```python
from build123d import *

# Parameters (mm, degrees)
SKETCH1_R              = 39
BOSS_EXTRUDE1_DEPTH    = 8
SKETCH2_R              = 8
BOSS_EXTRUDE2_DEPTH    = 10
SKETCH3_R              = 3
CUT_EXTRUDE1_DEPTH     = 59.017238817
M5_TAPPED_HOLE1_REACH  = 64.446
M5_TAPPED_HOLE1_BORE_R = 2.1
SKETCH5_W              = 8
SKETCH5_H              = 5


with BuildPart() as part:
    # Sketch1 → Boss-Extrude1 (new body)
    with BuildSketch(Plane.XY):
        Circle(SKETCH1_R)
    extrude(amount=BOSS_EXTRUDE1_DEPTH)

    # Sketch2 → Boss-Extrude2 (add)
    with BuildSketch(Plane.XY.offset(8)):
        Circle(SKETCH2_R)
    extrude(amount=BOSS_EXTRUDE2_DEPTH)

    # Sketch3 → Cut-Extrude1 (cut, through all)
    with BuildSketch(Plane.XY.offset(18)):
        Circle(SKETCH3_R)
    extrude(amount=-CUT_EXTRUDE1_DEPTH, mode=Mode.SUBTRACT)

    # M5 Tapped Hole1 bore (on position points) → M5 Tapped Hole1 (cut, up to next)
    with BuildSketch(Plane(origin=(-0.006341918, 7.999997486, 13), x_dir=(0.999999685782, 0.000792739743, 0), z_dir=(-0.000792739743, 0.999999685782, 0)), mode=Mode.PRIVATE) as m5_tapped_hole1_sk1:
        Circle(M5_TAPPED_HOLE1_BORE_R)
    m5_tapped_hole1_tool1 = extrude(m5_tapped_hole1_sk1.sketch, amount=-M5_TAPPED_HOLE1_REACH, mode=Mode.PRIVATE) & part.part
    add(m5_tapped_hole1_tool1.solids().sort_by_distance((-0.006342, 7.999997, 13))[0], mode=Mode.SUBTRACT)

    # Sketch5 → Cut-Revolve1 (revolve, cut)
    with BuildSketch(Plane(origin=(0, 0, 0), x_dir=(1, 0, 0), z_dir=(0, 1, 0))):
        with Locations((-39, -4)):
            Rectangle(SKETCH5_W, SKETCH5_H)
    revolve(axis=Axis((0, 0, 0), (0, 0, 1)), mode=Mode.SUBTRACT)


solid = part.part
```
Check sheet for the modelled part. Datum: model origin and axes. Units: mm. A direction names the side the tool comes from. Coordinates: 2 decimals unless noted, no trailing zeros. Loops run counter-clockwise (first coordinate to the right, second up) from the corner with the lowest first, then second, coordinate; pieces in that order, holes last.
1) Sectioned sample at C-C (x = 28). Record the boundary of the cut face in (y, z), and give its area (3 significant figures).
2) Access from +Z, -Z, +X, -X, +Y, -Y to the whole of each face (thin tool, end or side, straight path). Record for faces 4 (the face through (-1.73, -7.81, 12.93)), 5 (the face through (28, 21, 4)).
3) Sectioned sample at A-A (y = 0). Record the boundary of the cut face in (x, z), and give its area (3 significant figures).
4) Material ranges on probe 1 along Y at (x, z) = (0, 10.5); probe 2 along Z at (x, y) = (-22, -31.5); probe 3 along Y at (x, z) = (0, 4.25), recorded low to high.
5) Gauge pin test, flat ends, axial feed: pin 1 (10 mm diameter, centred on x = -17.5, y = -11.5, fed in from +Z); pin 2 (1.5 mm diameter, centred on x = 21.5, z = 6, fed in from +Y); pin 3 (2 mm diameter, centred on x = -7.5, z = 7, fed in from +Y); pin 4 (5 mm diameter, centred on x = 0, y = 0, fed in from -Z). Record the tip position at first contact, or that the pin passes through.
6) Release check for a two-part mould opening along Y. For faces 1 (the face through (-0.65, -2.93, 9.13)), 2 (the face through (32, -15, 6.5)), 3 (the face through (-5.077, 38.668, 0.74)) record: released by +Y, released by -Y, zero draft, split by the parting line, or undercut.
7) Sectioned sample at D-D (y = 24). Record the boundary of the cut face in (x, z).
8) Sectioned sample at B-B (x = 0). Count the separate pieces of the cut face and the enclosed holes in it, and give its area (3 significant figures).
Check sheet entries:
1. outline: (-27.15, 0) - (27.15, 0) - (27.15, 1.5) - (21, 1.5) - (21, 6.5) - (27.15, 6.5) - (27.15, 8) - (-27.15, 8) - (-27.15, 6.5) - (-21, 6.5) - (-21, 1.5) - (-27.15, 1.5) - close
1. area: 373 mm2
2. face 4: +Z
2. face 5: none
3. outline: (-39, 0) - (-3, 0) - (-3, 18) - (-8, 18) - (-8, 8) - (-39, 8) - (-39, 6.5) - (-35, 6.5) - (-35, 1.5) - (-39, 1.5) - close; (3, 0) - (39, 0) - (39, 1.5) - (35, 1.5) - (35, 6.5) - (39, 6.5) - (39, 8) - (8, 8) - (8, 18) - (3, 18) - close
3. area: 636 mm2
4. probe 1: y = -8 to -3, 3 to 8
4. probe 2: z = 0 to 1.5, 6.5 to 8
4. probe 3: y = -35 to -3, 3 to 35
5. pin 1: stops at z = 8
5. pin 2: stops at y = 32.9
5. pin 3: stops at y = 38.45
5. pin 4: passes through
6. face 1: undercut
6. face 2: zero draft
6. face 3: split by the parting line
7. outline: (-30.74, 0) - (30.74, 0) - (30.74, 1.5) - (25.48, 1.5) - (25.48, 6.5) - (30.74, 6.5) - (30.74, 8) - (-30.74, 8) - (-30.74, 6.5) - (-25.48, 6.5) - (-25.48, 1.5) - (-30.74, 1.5) - close
8. separate pieces: 3
8. enclosed holes: 0
8. area: 615 mm2
